from build123d import *

# Parameters (mm, degrees)
SKETCH5_W                    = 136
SKETCH5_H                    = 30
BASE_FLANGE1_DEPTH           = 1.5
EDGE_FLANGE1_STRIP_W         = 7
EDGE_FLANGE1_STRIP_H         = 1.5
EDGE_FLANGE1_STRIP_CUT_DEPTH = 30
EDGE_FLANGE1_DEPTH           = 30
SKETCH13_R                   = 2
CUT_EXTRUDE1_DEPTH           = 10
SKETCH14_W                   = 72.1
SKETCH14_H                   = 48.1
SKETCH14_R                   = 2
BOSS_EXTRUDE1_DEPTH          = 1.5
SKETCH15_R                   = 10
CUT_EXTRUDE2_DEPTH           = 10
FILLET1_R                    = 3
CUT_EXTRUDE5_DEPTH           = 10
FILLET4_R                    = 2
BOSS_EXTRUDE2_DEPTH          = 1.5


# Sheet-metal steps are written as plain solids
with BuildPart() as part:
    # Sketch5 → Base-Flange1 (new body)
    with BuildSketch(Plane(origin=(0, 0, 0), x_dir=(1, 0, 0), z_dir=(0, 1, 0))):
        with Locations((-68, 15)):
            Rectangle(SKETCH5_W, SKETCH5_H)
    extrude(amount=-BASE_FLANGE1_DEPTH)

    # Edge-Flange1 strip (across the edge) → Edge-Flange1 strip cut (cut)
    with BuildSketch(Plane(origin=(-136, 0, -30), x_dir=(1, 0, 0), z_dir=(0, 0, 1))):
        with Locations((-3, -0.75)):
            Rectangle(EDGE_FLANGE1_STRIP_W, EDGE_FLANGE1_STRIP_H)
    edge_flange1_strip_cut = extrude(amount=EDGE_FLANGE1_STRIP_CUT_DEPTH, mode=Mode.SUBTRACT)

    # Edge-Flange1 section (across the edge) → Edge-Flange1 (add)
    with BuildSketch(Plane(origin=(-136, 0, -30), x_dir=(1, 0, 0), z_dir=(0, 0, 1))):
        with BuildLine():
            Line((-1.5, 0.5), (-1.5, 65))
            Line((-1.5, 65), (0, 65))
            Line((0, 65), (0, 0.5))
            ThreePointArc((0, 0.5), (0.146446609, 0.146446609), (0.5, 0))
            Line((0.5, 0), (0.5, -1.5))
            ThreePointArc((0.5, -1.5), (-0.914213562, -0.914213562), (-1.5, 0.5))
        make_face()
    edge_flange1 = extrude(amount=EDGE_FLANGE1_DEPTH)

    # Sketch13 → Cut-Extrude1 (cut)
    with BuildSketch(Plane.ZY.offset(137.5)):
        with Locations(Location((-24, 61, 0), (0, 0, 270))):
            Circle(SKETCH13_R)
        with Locations(Location((-4, 61, 0), (0, 0, 270))):
            Circle(SKETCH13_R)
    cut_extrude1 = extrude(amount=-CUT_EXTRUDE1_DEPTH, mode=Mode.SUBTRACT)

    # Mirror1: Edge-Flange1 strip cut, Edge-Flange1, Cut-Extrude1 across plane
    add(edge_flange1_strip_cut.mirror(Plane(origin=(-68, 0, 0), x_dir=(0, 0, 1), z_dir=(1, 0, 0))), mode=Mode.SUBTRACT)
    add(edge_flange1.mirror(Plane(origin=(-68, 0, 0), x_dir=(0, 0, 1), z_dir=(1, 0, 0))))
    add(cut_extrude1.mirror(Plane(origin=(-68, 0, 0), x_dir=(0, 0, 1), z_dir=(1, 0, 0))), mode=Mode.SUBTRACT)

    # Sketch14 → Boss-Extrude1 (add)
    with BuildSketch(Plane.XZ.offset(1.5)):
        with Locations((-68, -12)):
            Rectangle(SKETCH14_W, SKETCH14_H)
        with Locations(Location((-100, 8, 0), (0, 0, 270))):
            Circle(SKETCH14_R, mode=Mode.SUBTRACT)
        with Locations(Location((-100, -32, 0), (0, 0, 90))):
            Circle(SKETCH14_R, mode=Mode.SUBTRACT)
        with Locations(Location((-36, -32, 0), (0, 0, 270))):
            Circle(SKETCH14_R, mode=Mode.SUBTRACT)
        with Locations(Location((-36, 8, 0), (0, 0, 90))):
            Circle(SKETCH14_R, mode=Mode.SUBTRACT)
    extrude(amount=-BOSS_EXTRUDE1_DEPTH)

    # Sketch15 → Cut-Extrude2 (cut)
    with BuildSketch(Plane.XZ.offset(1.5)):
        with Locations(Location((-68, -17, 0), (0, 0, 270))):
            Circle(SKETCH15_R)
    extrude(amount=-CUT_EXTRUDE2_DEPTH, mode=Mode.SUBTRACT)

    # Fillet1
    fillet1_edges = [part.edges().sort_by_distance(p)[0] for p in [
        (-31.95, -0.75, 0),
        (-104.05, -0.75, 0),
        (-104.05, -0.75, -30),
        (-104.05, -0.75, -36.05),
        (-31.95, -0.75, -30),
        (-104.05, -0.75, 12.05),
        (-31.95, -0.75, 12.05),
        (-31.95, -0.75, -36.05),
        (-136.75, 65, -30),
        (-136.75, 65, 0),
        (0.75, 65, 0),
        (0.75, 65, -30),
    ]]
    fillet(fillet1_edges, radius=FILLET1_R)

    # Sketch16 → Cut-Extrude5 (cut)
    with BuildSketch(Plane(origin=(0, 0, 0), x_dir=(1, 0, 0), z_dir=(0, 1, 0))):
        with BuildLine():
            ThreePointArc((-97.755689719, 28.628713693), (-97.827360667, 28.582085676), (-97.9, 28.536981086))
            Line((-97.9, 28.536981086), (-97.9, -3.694482809))
            Line((-97.9, -3.694482809), (-79.402624763, 10.756591595))
            ThreePointArc((-79.402624763, 10.756591595), (-80.917918539, 15.541445711), (-80.507682349, 20.543710239))
            Line((-80.507682349, 20.543710239), (-97.755689719, 28.628713693))
        make_face()
        with BuildLine():
            Line((-69.609347694, 29.9), (-90.572232827, 29.9))
            Line((-90.572232827, 29.9), (-78.725060069, 24.34663777))
            ThreePointArc((-78.725060069, 24.34663777), (-74.763457823, 28.102055588), (-69.609347694, 29.9))
        make_face()
        with BuildLine():
            Line((-57.274939931, 24.34663777), (-45.427767173, 29.9))
            Line((-45.427767173, 29.9), (-66.390652306, 29.9))
            ThreePointArc((-66.390652306, 29.9), (-61.236542177, 28.102055588), (-57.274939931, 24.34663777))
        make_face()
        with BuildLine():
            Line((-36, 36.05), (-99.999999884, 36.05))
            ThreePointArc((-99.999999884, 36.05), (-98.012853754, 35.528987078), (-96.536981086, 34.1))
            Line((-96.536981086, 34.1), (-39.463018914, 34.1))
            ThreePointArc((-39.463018914, 34.1), (-37.987146195, 35.528987107), (-36, 36.05))
        make_face()
        with BuildLine():
            Line((-38.1, -3.694482809), (-38.1, 28.536981086))
            ThreePointArc((-38.1, 28.536981086), (-38.172639333, 28.582085676), (-38.244310281, 28.628713693))
            Line((-38.244310281, 28.628713693), (-55.492317651, 20.543710239))
            ThreePointArc((-55.492317651, 20.543710239), (-55.123667631, 18.788872475), (-55, 17))
            ThreePointArc((-55, 17), (-55.405673461, 13.777743176), (-56.597375237, 10.756591595))
            Line((-56.597375237, 10.756591595), (-38.1, -3.694482809))
        make_face()
        with BuildLine():
            ThreePointArc((-59.183080213, 7.446889225), (-68, 4), (-76.816919787, 7.446889225))
            Line((-76.816919787, 7.446889225), (-93.900937995, -5.9))
            Line((-93.900937995, -5.9), (-42.099062005, -5.9))
            Line((-42.099062005, -5.9), (-59.183080213, 7.446889225))
        make_face()
        with BuildLine():
            ThreePointArc((-96.536981086, -10.1), (-98.012853805, -11.528987107), (-100, -12.05))
            Line((-100, -12.05), (-36, -12.05))
            ThreePointArc((-36, -12.05), (-37.987146195, -11.528987107), (-39.463018914, -10.1))
            Line((-39.463018914, -10.1), (-96.536981086, -10.1))
        make_face()
    extrude(amount=-CUT_EXTRUDE5_DEPTH, mode=Mode.SUBTRACT)

    # Fillet4
    fillet4_edges = [part.edges().sort_by_distance(p)[0] for p in [
        (-56.597375237, -0.75, -10.756591595),
        (-55.492317651, -0.75, -20.543710239),
        (-38.1, -0.75, 3.694482809),
        (-39.463018914, -0.75, -34.1),
        (-96.536981086, -0.75, -34.1),
        (-57.274939931, -0.75, -24.34663777),
        (-66.390652306, -0.75, -29.9),
        (-45.427767173, -0.75, -29.9),
        (-69.609347694, -0.75, -29.9),
        (-78.725060069, -0.75, -24.34663777),
        (-90.572232827, -0.75, -29.9),
        (-76.816919787, -0.75, -7.446889225),
        (-59.183080213, -0.75, -7.446889225),
        (-42.099062005, -0.75, 5.9),
        (-93.900937995, -0.75, 5.9),
        (-96.536981086, -0.75, 10.1),
        (-39.463018914, -0.75, 10.1),
        (-80.507682349, -0.75, -20.543710239),
        (-79.402624763, -0.75, -10.756591595),
        (-97.9, -0.75, 3.694482809),
    ]]
    fillet(fillet4_edges, radius=FILLET4_R)

    # Sketch17 → Boss-Extrude2 (add)
    with BuildSketch(Plane(origin=(0, 0, 0), x_dir=(1, 0, 0), z_dir=(0, 1, 0))):
        with BuildLine():
            Line((-97.9, 28.536981086), (-97.9, 23.976872191))
            ThreePointArc((-97.9, 23.976872191), (-96.509362469, 26.50866058), (-93.626698371, 26.693248999))
            Line((-93.626698371, 26.693248999), (-97.755689719, 28.628713693))
            ThreePointArc((-97.755689719, 28.628713693), (-97.827360667, 28.582085676), (-97.9, 28.536981086))
        make_face()
        with BuildLine():
            Line((-38.244310281, 28.628713693), (-42.373301629, 26.693248999))
            ThreePointArc((-42.373301629, 26.693248999), (-39.490637531, 26.50866058), (-38.1, 23.976872191))
            Line((-38.1, 23.976872191), (-38.1, 28.536981086))
            ThreePointArc((-38.1, 28.536981086), (-38.172639333, 28.582085676), (-38.244310281, 28.628713693))
        make_face()
    extrude(amount=-BOSS_EXTRUDE2_DEPTH)


solid = part.part
Input: part model. Units: mm. Frame: model coordinates. A direction names the side the tool comes from. Give positions to 0.01 mm unless a question says otherwise; leave off trailing zeros. Write each loop counter-clockwise with the first axis right and the second up, starting at its lowest first coordinate (ties: lowest second). Pieces come first, ordered by that corner, then holes. Notation, with made-up numbers: (-30.5, -18.75) -> (-0.5, -18.75) arc R22 cw to (-0.5, 5.25) -> close; hole circle Ø2 at (4.25, 71.25). An arc over 180 degrees is marked (long way). Use one line per item in the form item = value. Start each with the question number.
1) Ray query, probe 1 along Z at (x, y) = (-36, -0.6); probe 2 along X at (y, z) = (56.5, -28.5); probe 3 along Z at (x, y) = (1, 61). Return the intervals inside material, ascending. Write a range as from..to.
2) Section query A-A on y = 14.5. Return the cut outline in (x, z).
3) Pin query (flat end, axial travel): pin 1 (1.2 mm diameter, centred on x = -55.5, y = -0.5, fed in from +Z); pin 2 (1.6 mm diameter, centred on y = -1, z = 5.5, fed in from +X); pin 3 (1.2 mm diameter, centred on y = -1, z = -17.5, fed in from +X); pin 4 (6.5 mm diameter, centred on y = 61, z = -24, fed in from +X). Return the tip coordinate at first contact, or that it passes through.
4) Section query B-B on x = -21. Return the cut outline in (y, z), then the cut area to 3 significant figures.
5) Draft query along Y for faces 1 (the cylindrical face through (-137, 63, -4)), 2 (the cylindrical face through (-39.526, -0.74, -26.531)), 3 (the cylindrical face through (0.74, 64.1, -29.14)), 4 (the cylindrical face through (1, 63, -24)). Return one class per face: pulls with the +Y half, pulls with the -Y half, needs draft (parallel to the pull), parting line crosses it, or undercut.
6) Set-up query: faces 5 (the cylindrical face through (-96.54, -0.74, -26.49)), 6 (the flat face through (-137, 16, -30)), 7 (the flat face through (-137, 16, 0)). Return all of +Z, -Z, +X, -X, +Y, -Y with unobstructed straight access to the full face (end or side cutting, diameter ignored); none if empty.
Outcome:
q1.probe_1 = -36.05..-34, -30..6, 10..12.05
q1.probe_2 = -137.5..-136, 0..1.5
q1.probe_3 = -30..-26, -22..-6, -2..0
q2.outline = (-137.5, -30) -> (-136, -30) -> (-136, 0) -> (-137.5, 0) -> close; (0, -30) -> (1.5, -30) -> (1.5, 0) -> (0, 0) -> close
q3.pin_1 = 10.1
q3.pin_2 = -31.95
q3.pin_3 = 1.29
q3.pin_4 = 1.5
q4.outline = (-1.5, -30) -> (0, -30) -> (0, 0) -> (-1.5, 0) -> close
q4.area = 45.0 mm^2
q5.face_1 = undercut
q5.face_2 = needs draft
q5.face_3 = pulls with the +Y half
q5.face_4 = undercut
q6.face_5 = +Y, -Y
q6.face_6 = -Z, -X, +Y, -Y
q6.face_7 = +Z, -X, +Y, -Y
